For this review, take the finished solid that the model builds, in its own axes (mm). Give positions to 0.01 mm unless a question says otherwise; leave off trailing zeros. Write each loop counter-clockwise with the first axis right and the second up, starting at its lowest first coordinate (ties: lowest second). Pieces come first, ordered by that corner, then holes. Notation, with made-up numbers: (27, 39) -> (73, 39) arc R19 cw to (73, 61) -> close; hole circle Ø5 at (58.25, 24). An arc over 180 degrees is marked (long way). Answer as CSV lines item,"result".
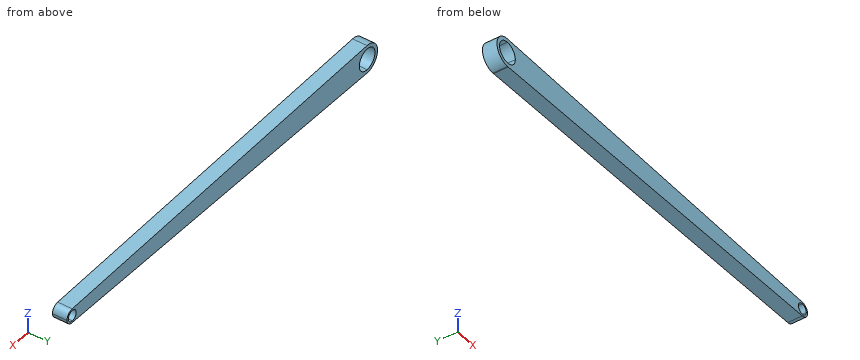
```python
from build123d import *

# Parameters (mm, degrees)
BOSS_EXTRUDE1_DEPTH = 64


with BuildPart() as part:
    # Sketch1 → Boss-Extrude1 (new body)
    with BuildSketch(Plane(origin=(0, 0, 0), x_dir=(1, 0, 0), z_dir=(0, 1, 0))):
        with BuildLine():
            ThreePointArc((64, 64), (45.254833996, 18.745166004), (0, 0))
            Line((0, 0), (1800, 0))
            ThreePointArc((1800, 0), (1768, 32), (1800, 64))
            Line((1800, 64), (4.545364872, 127.838387027))
            ThreePointArc((4.545364872, 127.838387027), (46.834300207, 107.618210923), (64, 64))
        make_face()
        with BuildLine():
            ThreePointArc((0, 128), (-64, 64), (0, 0))
            Line((0, 0), (0, 16))
            ThreePointArc((0, 16), (-48, 64), (0, 112))
            Line((0, 112), (0, 128))
        make_face()
        with BuildLine():
            Line((0, 16), (0, 0))
            ThreePointArc((0, 0), (45.254833996, 18.745166004), (64, 64))
            ThreePointArc((64, 64), (46.834300207, 107.618210923), (4.545364872, 127.838387027))
            Line((4.545364872, 127.838387027), (0, 128))
            Line((0, 128), (0, 112))
            ThreePointArc((0, 112), (33.941125497, 97.941125497), (48, 64))
            ThreePointArc((48, 64), (33.941125497, 30.058874503), (0, 16))
        make_face()
        with BuildLine():
            ThreePointArc((1800, 64), (1768, 32), (1800, 0))
            Line((1800, 0), (1800, 8))
            ThreePointArc((1800, 8), (1776, 32), (1800, 56))
            Line((1800, 56), (1800, 64))
        make_face()
        with BuildLine():
            Line((1800, 8), (1800, 0))
            ThreePointArc((1800, 0), (1822.627416998, 9.372583002), (1832, 32))
            ThreePointArc((1832, 32), (1822.627416998, 54.627416998), (1800, 64))
            Line((1800, 64), (1800, 56))
            ThreePointArc((1800, 56), (1816.970562748, 48.970562748), (1824, 32))
            ThreePointArc((1824, 32), (1816.970562748, 15.029437252), (1800, 8))
        make_face()
    extrude(amount=BOSS_EXTRUDE1_DEPTH)


solid = part.part
```
Q1. Add section C-C (x = 307). Write out the cut boundary in (y, z).
Answer block:
outline,"(0, -117.08) -> (64, -117.08) -> (64, 0) -> (0, 0) -> close"
Q2. Add section B-B (y = 42). Write out the cut boundary in (x, z), plus the area to 3 significant figures.
Answer block:
outline,"(0, -128) -> (1800, -64) arc R32 ccw to (1800, 0) -> (0, 0) arc R64 ccw to start; hole circle Ø96 at (0, -64); hole circle Ø48 at (1800, -32)"
area,"172,000 mm2"
Q3. Add section D-D (x = 844). Write out the cut boundary in (y, z), plus the area to 3 significant figures.
Answer block:
outline,"(0, -97.99) -> (64, -97.99) -> (64, 0) -> (0, 0) -> close"
area,"6,270 mm2"
Q4. Add section A-A (z = -90). Write out the cut boundary in (x, y), plus the area to 3 significant figures.
Answer block:
outline,"(-58.48, 0) -> (-40.35, 0) -> (-40.35, 64) -> (-58.48, 64) -> close; (40.35, 0) -> (1068.75, 0) -> (1068.75, 64) -> (40.35, 64) -> close"
area,"67,000 mm2"
Q5. Clearance check with flat-ended pins moving along their axes: pin 1 (4 mm diameter, centred on y = 38.5, z = -49.5, fed in from -X); pin 2 (2 mm diameter, centred on x = 1618, y = 9, fed in from -Z); pin 3 (10 mm diameter, centred on x = 1151, y = 46, fed in from -Z). State where each tip first meets the part, or that it passes through.
Answer block:
pin 1,"stops at x = -62.77"
pin 2,"stops at z = -70.51"
pin 3,"stops at z = -87.25"
Q6. To check wall thickness, follow probe 1 along X at (y, z) = (60, -39); probe 2 along X at (y, z) = (14.5, -12.5); probe 3 along X at (y, z) = (37.5, -53). State the ranges of each line that lie inside material, in increasing order. Write a range as [from, to].
Answer block:
probe 1,"x = [-58.92, -40.98], [40.98, 1777.04], [1822.96, 1831.22]"
probe 2,"x = [-38, 1786.01], [1813.99, 1825.37]"
probe 3,"x = [-63.05, -46.72], [46.72, 1788.38], [1811.62, 1824.15]"
